Here's how the part is built. I have some questions about the finished solid (model axes, mm). Round coordinates to 2 decimals unless told otherwise and drop trailing zeros. Write each loop counter-clockwise with the first axis right and the second up, starting at its lowest first coordinate (ties: lowest second). Pieces come first, ordered by that corner, then holes. Notation, with made-up numbers: M 7.25,-23 L 59.25,-23 A23 cw 59.25,4 Z; hole C 27.25,-5.75 d4. An arc over 180 degrees is marked long. Write item = value, one per line. Start each with the question number.
(1) I want a section at D-D (y = 2.5). List the corners of the cut face in (x, z) for me.
(2) Will these pins go through, and if not, where does the flat tip stop? pin 1 Ø1 at (y, z) = (-2, -18.5) entering from -X; pin 2 Ø0.9 at (x, z) = (0, 42.5) entering from +Y; pin 3 Ø1 at (y, z) = (4, 46) entering from -X.
(3) I want a section at B-B (z = 34). List the corners of the cut face in (x, y) for me, and give its area (3 significant figures).
(4) I need wall thicknesses on line 1 along X through (y, z) = (0.25, -17); line 2 along Z through (x, y) = (0.25, 4.75); line 3 along X through (y, z) = (3.5, 26). Which ranges of each line are inside material? Lowest first, please.
(5) I want a section at A-A (x = 0). List the corners of the cut face in (y, z) for me, and give its area (4 significant figures).
(6) I want a section at C-C (y = -1.75). List the corners of the cut face in (x, z) for me, and give its area (3 significant figures).
(7) If we mould it in two halves opening along X, with no side actions, what happens to faces 1 (the cylindrical face through (-1.08, -4.88, 0.71)), 2 (the flat face through (0, 0, 50.5)), 3 (the flat face through (0, 3.5, 43))? For each: released by +X, released by -X, zero draft, split by the parting line, or undercut.
```python
from build123d import *

# Parameters (mm, degrees)
SKETCH1_R           = 5
BOSS_EXTRUDE1_DEPTH = 50.5
CUT_EXTRUDE1_START  = 5
CUT_EXTRUDE1_DEPTH  = 1.5


with BuildPart() as part:
    # Sketch1 → Boss-Extrude1 (new, symmetric)
    with BuildSketch(Plane.XY):
        Circle(SKETCH1_R)
    extrude(amount=BOSS_EXTRUDE1_DEPTH, both=True)

    # Sketch2 → Cut-Extrude1 (cut)
    with BuildSketch(Plane(origin=(0, 0, 0), x_dir=(1, 0, 0), z_dir=(0, 1, 0)).offset(CUT_EXTRUDE1_START)):
        with BuildLine():
            Line((-1.5, -37), (-1.5, -50.5))
            Line((-1.5, -50.5), (1.5, -50.5))
            Line((1.5, -50.5), (1.5, -37))
            ThreePointArc((1.5, -37), (0, -35.5), (-1.5, -37))
        make_face()
    extrude(amount=-CUT_EXTRUDE1_DEPTH, mode=Mode.SUBTRACT)


solid = part.part
```
Returned:
q1.outline = M -4.33,-50.5 L 4.33,-50.5 L 4.33,50.5 L -4.33,50.5 Z
q2.pin_1 = -4.77
q2.pin_2 = 3.5
q2.pin_3 = -3.57
q3.outline = C 0,0 d10
q3.area = 78.5 mm²
q4.line_1 = -4.99 to 4.99
q4.line_2 = -50.5 to 35.52
q4.line_3 = -3.57 to 3.57
q5.outline = M -5,-50.5 L 5,-50.5 L 5,35.5 L 3.5,35.5 L 3.5,50.5 L -5,50.5 Z
q5.area = 987.5 mm²
q6.outline = M -4.68,-50.5 L 4.68,-50.5 L 4.68,50.5 L -4.68,50.5 Z
q6.area = 946 mm²
q7.face_1 = split by the parting line
q7.face_2 = zero draft
q7.face_3 = undercut
